The model under review builds one solid part; all positions refer to its coordinate system, in mm. Coordinates: 2 decimals unless noted, no trailing zeros. Order: outer loops, then holes, each group sorted by start corner. A loop starts at its lowest first (then second) coordinate and runs counter-clockwise, first axis right, second up.
from build123d import *

# Parameters (mm, degrees)
SKETCH1_R           = 3.25
BOSS_EXTRUDE1_DEPTH = 6
SKETCH2_R           = 4
CUT_EXTRUDE1_DEPTH  = 4
CHAMFER1_START      = -18.742104721
CHAMFER1_2_DEPTH    = 45.742104721
CHAMFER1_START_2    = -27
CHAMFER1_3_DEPTH    = 45.742104721
CHAMFER2_SIZE       = 1.2


with BuildPart() as part:
    # Sketch1 → Boss-Extrude1 (new body)
    with BuildSketch(Plane(origin=(0, 36, 0), x_dir=(1, 0, 0), z_dir=(0, 1, 0))):
        with BuildLine():
            Line((-60.898028106, -44.25832974), (60.898028106, -44.25832974))
            Line((60.898028106, -44.25832974), (79.111739679, -68.428741366))
            ThreePointArc((79.111739679, -68.428741366), (0, -104.6), (-79.111739679, -68.428741366))
            Line((-79.111739679, -68.428741366), (-60.898028106, -44.25832974))
        make_face()
        with Locations(Location((38.031910385, -62.101530721, 0), (0, 0, 270))):
            Circle(SKETCH1_R, mode=Mode.SUBTRACT)
        with Locations(Location((49.125752403, -76.823556322, 0), (0, 0, 270))):
            Circle(SKETCH1_R, mode=Mode.SUBTRACT)
        with Locations(Location((-49.125752403, -76.823556322, 0), (0, 0, 90))):
            Circle(SKETCH1_R, mode=Mode.SUBTRACT)
        with Locations(Location((-38.031910385, -62.101530721, 0), (0, 0, 90))):
            Circle(SKETCH1_R, mode=Mode.SUBTRACT)
    extrude(amount=BOSS_EXTRUDE1_DEPTH)

    # Sketch2 → Cut-Extrude1 (cut)
    with BuildSketch(Plane.XZ.offset(-36)):
        with Locations(Location((0, 91.29880712, 0), (0, 0, 270))):
            Circle(SKETCH2_R)
        with Locations(Location((0, 67.77856843, 0), (0, 0, 270))):
            Circle(SKETCH2_R)
        with Locations((0, 44.25832974)):
            Circle(SKETCH2_R)
    extrude(amount=-CUT_EXTRUDE1_DEPTH, mode=Mode.SUBTRACT)

    # Chamfer1: read off the stored shape, not the designer's step
    # Chamfer1 outline → Chamfer1 (revolve, cut)
    with BuildSketch(Plane.XY):
        Polygon((104.6, 37.2), (103.4, 36), (104.6, 36), align=None)
    revolve(axis=Axis((0, 0, 0), (0, 1, 0)), mode=Mode.SUBTRACT)

    # Chamfer1 2 outline → Chamfer1 2 (cut)
    with BuildSketch(Plane(origin=(0, 0, 0), x_dir=(0.9431059319759283, 0.23510763606464977, -0.23510763606464977), z_dir=(0.3324924075401055, -0.6668765998774377, 0.6668765998774377)).offset(CHAMFER1_START)):
        Polygon((46, 57.599737343), (-59.092758772, 57.599737343), (-81.95286654, 74.690799308), (-83, 75.473675007), (-83, 56), (46, 56), align=None)
    extrude(amount=CHAMFER1_2_DEPTH, mode=Mode.SUBTRACT)

    # Chamfer1 3 outline → Chamfer1 3 (cut)
    with BuildSketch(Plane(origin=(0, 0, 0), x_dir=(0.9431059319759302, -0.23510763606464624, 0.23510763606464624), z_dir=(0.33249240754010045, 0.6668765998774391, -0.6668765998774391)).offset(CHAMFER1_START_2)):
        Polygon((-45, -57.599737343), (59.092758772, -57.599737343), (81.95286654, -74.690799308), (83, -75.473675007), (83, -56), (-45, -56), align=None)
    extrude(amount=CHAMFER1_3_DEPTH, mode=Mode.SUBTRACT)

    # Chamfer2
    chamfer2_edges = [part.edges().sort_by_distance(p)[0] for p in [
        (70.004883892, 42, 56.343535553),
        (0, 42, 44.25832974),
        (-70.004883892, 42, 56.343535553),
        (0, 42, 104.6),
    ]]
    chamfer(chamfer2_edges, length=CHAMFER2_SIZE)


solid = part.part
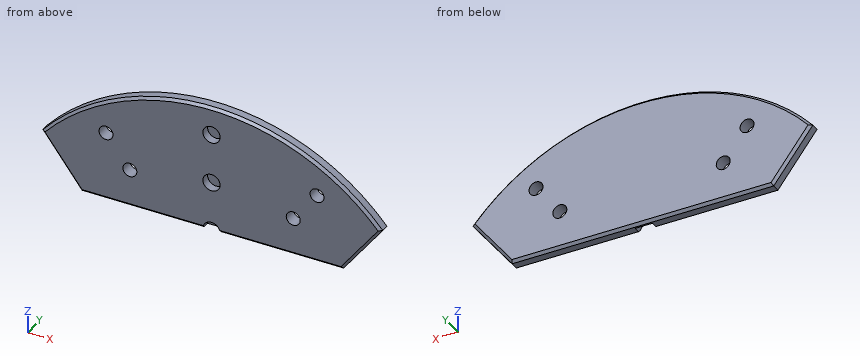
(1) Insertion check: pin 1 Ø4 at (x, z) = (1, 66.5) entering from -Y; pin 2 Ø1 at (x, y) = (42, 39) entering from +Z. Each pin has a flat end and moves straight along its axis. Give the tip position at first contact, or say it passes through.
(2) Consider section A-A (x = 0). Give the boundary of the cut face in (y, z).
(3) Wall thickness on line 1 (X direction, y = 41.55, z = 76); line 2 (X direction, y = 36.3, z = 60); line 3 (X direction, y = 39, z = 93.5): over which ranges is each line inside the solid? List them lowest first.
(4) Consider section B-B (y = 38.7). Give the boundary of the cut face in (x, z).
Findings:
1. pin 1: stops at y = 40
1. pin 2: stops at z = 96.02
2. outline: (36, 48.26) - (40, 48.26) - (40, 44.26) - (40.8, 44.26) - (42, 45.46) - (42, 103.4) - (40.8, 104.6) - (37.2, 104.6) - (36, 103.4) - (36, 95.3) - (40, 95.3) - (40, 87.3) - (36, 87.3) - (36, 71.78) - (40, 71.78) - (40, 63.78) - (36, 63.78) - close
3. line 1: x = -70.77 to -52.27, -45.98 to 45.98, 52.27 to 70.77
3. line 2: x = -71.63 to -40.51, -35.55 to 35.55, 40.51 to 71.63
3. line 3: x = -46.89 to -3.34, 3.34 to 46.89
4. outline: (-79.11, 68.43) - (-60.9, 44.26) - (-4, 44.26) arc R4 cw to (4, 44.26) - (60.9, 44.26) - (79.11, 68.43) arc R104.6 ccw to start; hole circle Ø6.5 at (-49.13, 76.82); hole circle Ø6.5 at (-38.03, 62.1); hole circle Ø8 at (0, 67.78); hole circle Ø8 at (0, 91.3); hole circle Ø6.5 at (38.03, 62.1); hole circle Ø6.5 at (49.13, 76.82)
